Source: CAD feature listing. Evaluate the final solid. Frame: model axes, mm. Coordinates: 2 decimals unless noted, no trailing zeros. Loops run counter-clockwise (first coordinate to the right, second up) from the corner with the lowest first, then second, coordinate; pieces in that order, holes last.
Item 1: Pin query (flat end, axial travel): pin 1 Ø2 at (x, z) = (-0.5, -15.5) entering from -Y; pin 2 Ø1 at (x, y) = (0, 10) entering from +Z; pin 3 Ø1.3 at (x, z) = (0, 16.5) entering from -Y; pin 4 Ø4 at (x, y) = (-2, 47.5) entering from -Z. Return the tip coordinate at first contact, or that it passes through.
Item 2: Section query B-B, the plane z = 0. Return the cut outline in (x, y).
Item 3: Section query A-A, the plane x = -0.25. Return the cut outline in (y, z).
Item 4: Line query: probe 1 along X at (y, z) = (70, -7); probe 2 along X at (y, z) = (61, 15.5); probe 3 along Z at (x, y) = (-3.25, 31). Output: solid intervals per line, ascending.
Item 5: Section query C-C, the plane y = 43.5. Return the cut outline in (x, z), then the cut area to 3 significant figures.
Item 6: Section query D-D, the plane x = -5. Return the cut outline in (y, z).
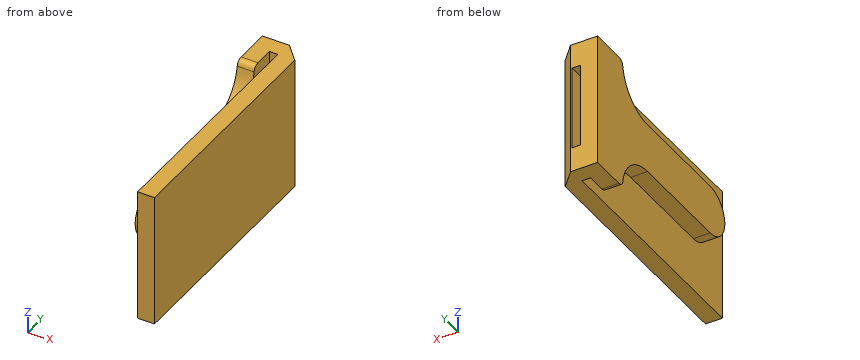
Autodesk Inventor part; units mm, degrees
ref_plane "YZ Plane" through (0, 0, 0) normal (1, 0, 0) x (0, 1, 0)
ref_plane "XZ Plane" through (0, 0, 0) normal (0, 1, 0) x (-1, 0, 0)
ref_plane "XY Plane" through (0, 0, 0) normal (0, 0, 1) x (1, 0, 0)
sketch "Sketch1" plane through (0, 0, 0) normal (0, 1, 0) x (-1, 0, 0)
  line L0 (-1.27, -12.7) -> (1.27, -12.7)
  line L1 (1.27, -12.7) -> (1.27, 12.7)
  line L2 (1.27, 12.7) -> (-1.27, 12.7)
  line L3 (-1.27, 12.7) -> (-1.27, -12.7)
  line L4 (-1.27, -12.7) -> (1.27, 12.7) construction
  line L5 (1.27, -12.7) -> (-1.27, 12.7) construction
  line L6 (-6.35, -20.1281) -> (6.35, -20.1281)
  line L7 (6.35, -20.1281) -> (6.35, 20.1281)
  line L8 (6.35, 20.1281) -> (-6.35, 20.1281)
  line L9 (-6.35, 20.1281) -> (-6.35, -20.1281)
  line L10 (-6.35, -20.1281) -> (6.35, 20.1281) construction
  line L11 (6.35, -20.1281) -> (-6.35, 20.1281) construction
  point P0 (0, 0)
  dimension "d0" = 2.54
  dimension "d1" = 25.4
  dimension "d2" = 12.7
extrude "Extrusion1" add sketch "Sketch1" along normal blind 76.2
sketch "Sketch2" plane through (-6.35, 0, 20.1281) normal (0, 0, 1) x (1, 0, 0)
  line L0 (5.08, 0) -> (5.08, 76.2)
  line L1 (7.62, 0) -> (7.62, 76.2)
  line L2 (0, 0) -> (12.7, 0)
  line L3 (0, 76.2) -> (12.7, 76.2)
  line L4 (5.08, 0) -> (5.08, 76.2)
  line L5 (5.08, 71.2) -> (7.62, 71.2)
  line L6 (8.12, 76.2) -> (12.7, 71.2)
  line L7 (12.7, 0) -> (12.7, 76.2)
  point P0 (6.35, 0)
  dimension "d5" = 5
  dimension "d6" = 0.5
  dimension "d7" = 5
extrude "Extrusion2" cut sketch "Sketch2" against normal through all contours L0 L5 L1 L2 | L6 L3 L7
sketch "Sketch3" plane through (-6.35, 0, -20.1281) normal (-1, 0, 0) x (0, 0, 1)
  line L0 (40.2562, 0) -> (40.2562, 71.2)
  arc A0 (40.2562, 63.5) -> (27.5562, 50.8) centre (40.2562, 50.8) ccw
  line L1 (27.5562, 50.8) -> (27.5562, 19.05)
  line L2 (0, 76.2) -> (40.2562, 76.2)
  arc A1 (12.7, 19.05) -> (27.5562, 19.05) centre (20.1281, 19.05) ccw
  line L3 (0, 0) -> (0, 76.2)
  arc A2 (12.7, 50.8) -> (0, 63.5) centre (0, 50.8) ccw
  line L4 (12.7, 19.05) -> (12.7, 50.8)
  line L5 (0, 0) -> (40.2562, 0)
  point P0 (20.1281, 0)
  point P1 (20.1281, 0)
  dimension "d10" = 12.7
  dimension "d11" = 25.4
  dimension "d13" = 19.05
extrude "Extrusion3" cut sketch "Sketch3" against normal up to surface (5.08 mm away)
fillet "Fillet1" radius 2 2 edges at (-3.81, 63.5, 20.1281) (-3.81, 63.5, -20.1281)
properties part number "Glass Slide Gripper"
Verdict:
1. pin 1: stops at y = 62.36
1. pin 2: passes through
1. pin 3: stops at y = 71.2
1. pin 4: stops at z = -7.43
2. outline: (-6.35, 11.62) - (-1.27, 11.62) - (-1.27, 76.2) - (-6.35, 76.2) - close; (1.27, 0) - (6.35, 0) - (6.35, 71.2) - (1.77, 76.2) - (1.27, 76.2) - close
3. outline: (71.2, -20.13) - (76.2, -20.13) - (76.2, -12.7) - (71.2, -12.7) - close; (71.2, 12.7) - (76.2, 12.7) - (76.2, 20.13) - (71.2, 20.13) - close
4. probe 1: x = -6.35 to -1.27, 1.27 to 6.35
4. probe 2: x = 1.27 to 6.35
4. probe 3: z = -7.43 to 7.43
5. outline: (-6.35, -7.43) - (-1.27, -7.43) - (-1.27, 7.43) - (-6.35, 7.43) - close; (1.27, -20.13) - (6.35, -20.13) - (6.35, 20.13) - (1.27, 20.13) - close
5. area: 280 mm2
6. outline: (19.05, -7.43) - (50.8, -7.43) arc R12.7 cw to (63.38, -18.4) arc R2 ccw to (65.36, -20.13) - (76.2, -20.13) - (76.2, 20.13) - (65.36, 20.13) arc R2 ccw to (63.38, 18.4) arc R12.7 cw to (50.8, 7.43) - (19.05, 7.43) arc R7.43 ccw to start
